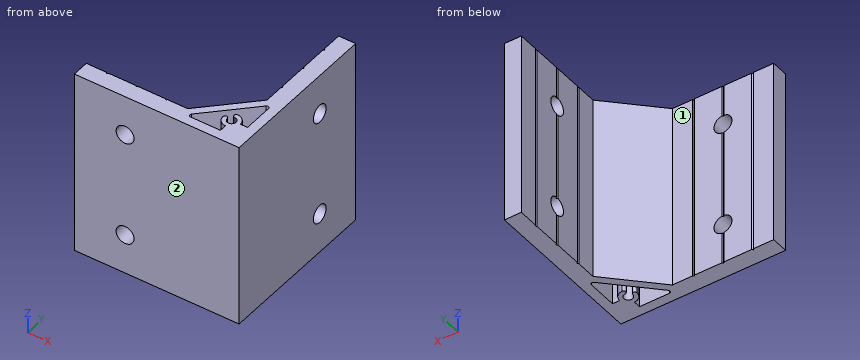
from build123d import *

# Parameters (mm, degrees)
EXTRUDE_1_DEPTH     = 44
SKETCH_2_R          = 4.25
CUT_EXTRUDE_1_DEPTH = 9
SKETCH_3_R          = 4.25
CUT_EXTRUDE_2_DEPTH = 9


with BuildPart() as part:
    # Эскиз1 → Бобышка-Вытянуть1 (new body, symmetric)
    with BuildSketch(Plane.XY):
        Polygon((-78, 0), (0, 0), (0, 78), (-8, 78), (-8, 68.5), (-7.5, 68), (-8, 67.5), (-8, 54.5), (-7.5, 54), (-8, 53.5), (-8, 40.5), (-7.5, 40), (-8, 39.5), (-8, 30), (-30, 8), (-39.5, 8), (-40, 7.5), (-40.5, 8), (-53.5, 8), (-54, 7.5), (-54.5, 8), (-67.5, 8), (-68, 7.5), (-68.5, 8), (-78, 8), align=None)
        with BuildLine():
            Line((-4.5, 12), (-4.5, 26.136038969))
            ThreePointArc((-4.5, 26.136038969), (-5.117316568, 27.059918502), (-6.207106781, 26.843145751))
            Line((-6.207106781, 26.843145751), (-26.843145751, 6.207106781))
            ThreePointArc((-26.843145751, 6.207106781), (-27.059918502, 5.117316568), (-26.136038969, 4.5))
            Line((-26.136038969, 4.5), (-12, 4.5))
            Line((-12, 4.5), (-12, 7.9))
            ThreePointArc((-12, 7.9), (-14.899137803, 9.100862197), (-16.1, 12))
            ThreePointArc((-16.1, 12), (-15.1, 13), (-14.1, 12))
            ThreePointArc((-14.1, 12), (-10.51507576, 10.51507576), (-12, 14.1))
            ThreePointArc((-12, 14.1), (-13, 15.1), (-12, 16.1))
            ThreePointArc((-12, 16.1), (-9.100862197, 14.899137803), (-7.9, 12))
            Line((-7.9, 12), (-4.5, 12))
        make_face(mode=Mode.SUBTRACT)
    extrude(amount=EXTRUDE_1_DEPTH, both=True)

    # Эскиз2 → Вырез-Вытянуть1 (cut, through all)
    with BuildSketch(Plane.ZY.offset(8)):
        with Locations(Location((-25, 54, 0), (0, 0, 270))):  # turned: the seam where the file's is
            Circle(SKETCH_2_R)
        with Locations(Location((25, 54, 0), (0, 0, 270))):  # turned: the seam where the file's is
            Circle(SKETCH_2_R)
    extrude(amount=-CUT_EXTRUDE_1_DEPTH, mode=Mode.SUBTRACT)

    # Эскиз3 → Вырез-Вытянуть2 (cut, through all)
    with BuildSketch(Plane(origin=(0, 8, 0), x_dir=(1, 0, 0), z_dir=(0, 1, 0))):
        with Locations(Location((-54, -25, 0), (0, 0, 180))):  # turned: the seam where the file's is
            Circle(SKETCH_3_R)
        with Locations(Location((-54, 25, 0), (0, 0, 180))):  # turned: the seam where the file's is
            Circle(SKETCH_3_R)
    extrude(amount=-CUT_EXTRUDE_2_DEPTH, mode=Mode.SUBTRACT)


solid = part.part
Check sheet for the modelled part. Datum: model origin and axes. Units: mm. Face numbers are marked on the shaded views. A direction names the side the tool comes from. Round coordinates to 2 decimals unless told otherwise and drop trailing zeros. Loops run counter-clockwise (first coordinate to the right, second up) from the corner with the lowest first, then second, coordinate; pieces in that order, holes last. Notation, with made-up numbers: (31.5, 57.5) -> (50.5, 57.5) arc R21 ccw to (50.5, 84.5) -> close; hole circle Ø6 at (43.5, 61). An arc over 180 degrees is marked (long way). Put each result on its own line as item: value. Start each with the question number.
1. Scan lines: probe 1 along Y at (x, z) = (-5.5, -25); probe 2 along Z at (x, y) = (-54, 3.5); probe 3 along Y at (x, z) = (-2.75, -25). Record each from-to range of solid material in increasing order.
2. Section check B-B (z = -25). Give the number of separate pieces and of enclosed holes in the cut face, plus the area to 3 significant figures.
3. Gauge pin test, flat ends, axial feed: pin 1 (4 mm diameter, centred on x = -19, z = -17, fed in from +Y); pin 2 (5 mm diameter, centred on x = -54, z = 25, fed in from -Y); pin 3 (5 mm diameter, centred on y = 60, z = 20.5, fed in from -X); pin 4 (1.5 mm diameter, centred on x = -64, z = 0.5, fed in from +Y). Record the tip position at first contact, or that the pin passes through.
4. Section check C-C (y = 22.5). Enter the section's corners in (x, z).
5. Section check A-A (x = -18.5). Enter the section's corners in (y, z), plus the area to 3 significant figures.
6. Access from +Z, -Z, +X, -X, +Y, -Y to the whole of each face (thin tool, end or side, straight path). Record for the marked faces 1 and 2.
7. Section check D-D (y = 63.5). Enter the section's corners in (x, z), plus the area to 3 significant figures.
Findings:
1. probe 1: y = 0 to 12, 27.14 to 49.75, 58.25 to 78
1. probe 2: z = -44 to -29.25, -20.75 to 20.75, 29.25 to 44
1. probe 3: y = 0 to 49.75, 58.25 to 78
2. separate pieces: 3
2. enclosed holes: 1
2. area: 1,080 mm^2
3. pin 1: stops at y = 21
3. pin 2: passes through
3. pin 3: stops at x = -8
3. pin 4: stops at y = 8
4. outline: (-15.5, -44) -> (-10.55, -44) -> (-10.55, 44) -> (-15.5, 44) -> close; (-4.5, -44) -> (0, -44) -> (0, 44) -> (-4.5, 44) -> close
5. outline: (0, -44) -> (4.5, -44) -> (4.5, 44) -> (0, 44) -> close; (14.55, -44) -> (19.5, -44) -> (19.5, 44) -> (14.55, 44) -> close
5. area: 832 mm^2
6. face 1: +Z, -Z, -X, +Y
6. face 2: +Z, -Z, +X, -X, -Y
7. outline: (-8, -44) -> (0, -44) -> (0, 44) -> (-8, 44) -> close
7. area: 704 mm^2
